from build123d import *

# Parameters (mm, degrees)
F0_R     = 25
F0_R_2   = 11.45
F1_DEPTH = 13
F2_R     = 25
F2_R_2   = 21
F2_R_3   = 11.45
F3_DEPTH = 6
F4_R     = 21
F4_R_2   = 11.45
F5_DEPTH = 2


with BuildPart() as f1:
    # F0 (on Front) → F1 (new body)
    with BuildSketch(Plane.XZ):
        Circle(F0_R)
        Circle(F0_R_2, mode=Mode.SUBTRACT)
    extrude(amount=F1_DEPTH)

    # F2 (on face) → F3 (cut)
    with BuildSketch(Plane.XZ.offset(13)):
        Circle(F2_R)
        Circle(F2_R_2, mode=Mode.SUBTRACT)
        Circle(F2_R_3)
    extrude(amount=-F3_DEPTH, mode=Mode.SUBTRACT)

    # F4 (on face) → F5 (cut)
    with BuildSketch(Plane(origin=(0, 0, 0), x_dir=(-1, 0, 0), z_dir=(0, 1, 0))):
        Circle(F4_R)
        Circle(F4_R_2, mode=Mode.SUBTRACT)
    extrude(amount=-F5_DEPTH, mode=Mode.SUBTRACT)


solid = f1.part
Model file for the job. Use its own axes, mm. A direction names the side the tool comes from. Give positions to 0.01 mm unless a question says otherwise; leave off trailing zeros. Order: outer loops, then holes, each group sorted by start corner. A loop starts at its lowest first (then second) coordinate and runs counter-clockwise, first axis right, second up. Notation, with made-up numbers: (-11.5, 76.5) - (12.5, 76.5) arc R17 cw to (12.5, 93.5) - close; hole circle Ø2 at (-37.75, 62.25). An arc over 180 degrees is marked (long way). Return JSON: item names as keys, results as strings.
1) Cut at D-D, the plane z = -18. Give the cut face in (x, y), plus the area to 3 significant figures.
Geometry says:
{"outline": "(-17.35, -7) - (-10.82, -7) - (-10.82, -13) - (10.82, -13) - (10.82, -7) - (17.35, -7) - (17.35, 0) - (10.82, 0) - (10.82, -2) - (-10.82, -2) - (-10.82, 0) - (-17.35, 0) - close", "area": "329 mm²"}
2) Cut at A-A, the plane x = 0. Give the cut face in (y, z), plus the area to 3 significant figures.
Geometry says:
{"outline": "(-13, -21) - (-7, -21) - (-7, -25) - (0, -25) - (0, -21) - (-2, -21) - (-2, -11.45) - (-13, -11.45) - close; (-13, 11.45) - (-2, 11.45) - (-2, 21) - (0, 21) - (0, 25) - (-7, 25) - (-7, 21) - (-13, 21) - close", "area": "266 mm²"}
3) Cut at B-B, the plane z = 0. Give the cut face in (x, y), plus the area to 3 significant figures.
Geometry says:
{"outline": "(-25, -7) - (-21, -7) - (-21, -13) - (-11.45, -13) - (-11.45, -2) - (-21, -2) - (-21, 0) - (-25, 0) - close; (11.45, -13) - (21, -13) - (21, -7) - (25, -7) - (25, 0) - (21, 0) - (21, -2) - (11.45, -2) - close", "area": "266 mm²"}
4) Cut at C-C, the plane y = -9.25. Give the cut face in (x, z).
Geometry says:
{"outline": "circle Ø42 at (0, 0); hole circle Ø22.9 at (0, 0)"}
5) Probe line 1 (Z direction, x = 0, y = -3.5); line 2 (Z direction, x = 0, y = -10); line 3 (Y direction, x = 12, z = 18). List the from-to ranges inside material, lowest first. Write a range as from..to.
Geometry says:
{"line 1": "-25..-11.45, 11.45..25", "line 2": "-21..-11.45, 11.45..21", "line 3": "-7..0"}
6) Pull direction X, two halves, no side cores. Call faces 1 (the flat face through (9, -13, -9)), 2 (the cylindrical face through (-2.48, -7.42, -11.18)), 3 (the cylindrical face through (20.03, -10.04, 6.31)), 4 (the flat face through (-9, -2, -9)): pulls with the +X half, pulls with the -X half, needs draft (parallel to the pull), parting line crosses it, or undercut.
Geometry says:
{"face 1": "needs draft", "face 2": "undercut", "face 3": "parting line crosses it", "face 4": "undercut"}
7) 3-axis set-ups, long thin cutter, end or side, ignore diameter. For faces 5 (the cylindrical face through (-20.03, -0.99, 6.31)), 6 (the cylindrical face through (23.846, -3.451, 7.509)), 7 (the flat face through (-5.7, -7, 20.5)): which of +Z, -Z, +X, -X, +Y, -Y reach the whole face in a straight line?
Geometry says:
{"face 5": "+Y", "face 6": "+Y, -Y", "face 7": "-Y"}
8) Flat gauge pins, fed straight in: P1, Ø6, axis at x = -4.5, z = 4.5, coming from the +Y side; P2, Ø6, axis at x = 13, z = -14, coming from the +Y side; P3, Ø1, axis at x = 1, y = -4, coming from the -Z side (3 decimals). Where does each tip first touch, or does it go through?
Geometry says:
{"P1": "through", "P2": "y = 0", "P3": "z = -24.995"}
